Could you check a few things on this model? Use its own coordinates, in mm. A direction names the side the tool comes from. Coordinates: 2 decimals unless noted, no trailing zeros. Write each loop counter-clockwise with the first axis right and the second up, starting at its lowest first coordinate (ties: lowest second). Pieces come first, ordered by that corner, then holes. Notation, with made-up numbers: M 51,36 L 82,36 A23 cw 82,47 Z; hole C 49,-9 d2. An arc over 180 degrees is marked long. Answer as CSV lines item,"result". Start each with the question number.
Item 1: I'm going to push flat-ended pins straight in: P1, Ø3, axis at x = -5.5, z = 0, coming from the +Y side; P2, Ø2, axis at x = 0, y = 1, coming from the +Z side; P3, Ø3, axis at y = 7, z = -8, coming from the +X side; P4, Ø2.5, axis at x = 0, y = 3.5, coming from the -Z side. Where does each tip first touch, or does it pass through?
Item 2: Suppose I cut it at A-A, the plane y = 5. Write out the boundary of the cut face in (x, z).
Item 3: On a 3-axis mill with a long thin cutter (end or side, diameter ignored), from which of +Z, -Z, +X, -X, +Y, -Y can I reach the whole of each face in a straight line? I mean faces 5 (the cylindrical face through (4.28, 7.77, -0.27)), 6 (the flat face through (1.3, 3.2, 8.3)), 7 (the flat face through (-8, 7, -5)). Say none if no direction works.
Item 4: If I drill on line 1 along X through (y, z) = (7.75, 0); line 2 along Y through (x, z) = (7.5, 4.25); line 3 along X through (y, z) = (0.6, 0), over which ranges is the centre line in solid material (lowest first)? Write a range as [from, to].
Item 5: We'd pull the mould along Y, two halves only. Please class faces 1 (the cylindrical face through (8.054, 5.462, 1.788)), 2 (the flat face through (-4, 0, 0)), 3 (the cylindrical face through (-6.3, 7.51, -8.21)), 4 (the cylindrical face through (8.054, 2.362, 1.788)): +Y half, -Y half, draft (parallel to the pull), parting line (faces both ways), or undercut.
Item 6: Suppose I cut it at B-B, the plane z = 0. State how many separate pieces and enclosed holes the cut face has, and give its area (3 significant figures).
```python
from build123d import *

# Parameters (mm, degrees)
SKETCH_1_R          = 11
EXTRUDE_1_DEPTH     = 9
SKETCH_2_R          = 0.5
CUT_EXTRUDE_1_DEPTH = 18.972200756
SKETCH_3_R          = 16.549134696
SKETCH_3_R_2        = 9.25
CUT_EXTRUDE_2_DEPTH = 7
SKETCH_4_W          = 2
SKETCH_4_H          = 1.7
SKETCH_5_W          = 5
SKETCH_5_H          = 6
CUT_EXTRUDE_3_DEPTH = 7
SKETCH_6_R          = 1.4
CUT_EXTRUDE_4_DEPTH = 7
SKETCH_7_R          = 1.25
CUT_EXTRUDE_5_DEPTH = 2.5
CUT_EXTRUDE_START   = -1.5
SKETCH_8_R          = 1.25
CUT_EXTRUDE_6_DEPTH = 1.5
SKETCH_9_W          = 7
SKETCH_9_H          = 8
SKETCH_9_W_2        = 5
SKETCH_9_H_2        = 6
CUT_EXTRUDE_7_DEPTH = 2
CHAMFER_1_SIZE      = 0.5
SKETCH_10_R         = 12.5
SKETCH_10_R_2       = 10.35
CUT_EXTRUDE_8_DEPTH = 10
FILLET_1_R          = 1
SKETCH_11_R         = 1.953999565
EXTRUDE_2_DEPTH     = 2


with BuildPart() as part:
    # 草图1 → 凸台-拉伸1 (new body)
    with BuildSketch(Plane(origin=(0, 0, 0), x_dir=(1, 0, 0), z_dir=(0, 1, 0))):
        with Locations(Location((0, 0, 0), (0, 0, 270))):
            Circle(SKETCH_1_R)
    extrude(amount=EXTRUDE_1_DEPTH)

    # 草图2 → 切除-拉伸1 (cut, through all)
    with BuildSketch(Plane(origin=(0, 9, 0), x_dir=(1, 0, 0), z_dir=(0, 1, 0))):
        with Locations(Location((-5.5, 0, 0), (0, 0, 270))):
            Circle(SKETCH_2_R)
        with Locations(Location((5.5, 0, 0), (0, 0, 270))):
            Circle(SKETCH_2_R)
    extrude(amount=-CUT_EXTRUDE_1_DEPTH, mode=Mode.SUBTRACT)

    # 草图3 → 切除-拉伸2 (cut)
    with BuildSketch(Plane.XZ):
        Circle(SKETCH_3_R)
        with Locations(Location((0, 0, 0), (0, 0, 270))):
            Circle(SKETCH_3_R_2, mode=Mode.SUBTRACT)
    extrude(amount=-CUT_EXTRUDE_2_DEPTH, mode=Mode.SUBTRACT)

    # 草图4 → 切除-旋转1 (revolve, cut)
    with BuildSketch(Plane.XY, mode=Mode.PRIVATE) as cut_revolve_1_sk:
        with Locations((-9.25, 5.45)):
            Rectangle(SKETCH_4_W, SKETCH_4_H)
        with Locations((-9.25, 2.35)):
            Rectangle(SKETCH_4_W, SKETCH_4_H)
    revolve(cut_revolve_1_sk.sketch.rotate(Axis((0, 0, 0), (0, 1, 0)), 270), axis=Axis((0, 0, 0), (0, 1, 0)), mode=Mode.SUBTRACT)

    # 草图5 → 切除-拉伸3 (cut)
    with BuildSketch(Plane.XZ):
        Rectangle(SKETCH_5_W, SKETCH_5_H)
    extrude(amount=-CUT_EXTRUDE_3_DEPTH, mode=Mode.SUBTRACT)

    # 草图6 → 切除-拉伸4 (cut)
    with BuildSketch(Plane(origin=(0, 9, 0), x_dir=(1, 0, 0), z_dir=(0, 1, 0))):
        with Locations(Location((0, 0, 0), (0, 0, 270))):
            Circle(SKETCH_6_R)
    extrude(amount=-CUT_EXTRUDE_4_DEPTH, mode=Mode.SUBTRACT)

    # 草图7 → 切除-拉伸5 (cut)
    with BuildSketch(Plane(origin=(0, 9, 0), x_dir=(1, 0, 0), z_dir=(0, 1, 0))):
        with Locations(Location((-5.5, 0, 0), (0, 0, 270))):
            Circle(SKETCH_7_R)
        with Locations(Location((5.5, 0, 0), (0, 0, 270))):
            Circle(SKETCH_7_R)
    extrude(amount=-CUT_EXTRUDE_5_DEPTH, mode=Mode.SUBTRACT)

    # 草图8 → 切除-拉伸6 (cut)
    with BuildSketch(Plane.XZ.offset(CUT_EXTRUDE_START)):
        with Locations(Location((-5.5, 0, 0), (0, 0, 90))):
            Circle(SKETCH_8_R)
        with Locations(Location((5.5, 0, 0), (0, 0, 90))):
            Circle(SKETCH_8_R)
    extrude(amount=CUT_EXTRUDE_6_DEPTH, mode=Mode.SUBTRACT)

    # 草图9 → 切除-拉伸7 (cut)
    with BuildSketch(Plane.XZ):
        Rectangle(SKETCH_9_W, SKETCH_9_H)
        Rectangle(SKETCH_9_W_2, SKETCH_9_H_2, mode=Mode.SUBTRACT)
    extrude(amount=-CUT_EXTRUDE_7_DEPTH, mode=Mode.SUBTRACT)

    # 倒角1
    chamfer_1_edges = [part.edges().sort_by_distance(p)[0] for p in [
        (0, 0, 9.25),
    ]]
    chamfer(chamfer_1_edges, length=CHAMFER_1_SIZE)

    # 草图10 → 切除-拉伸8 (cut)
    with BuildSketch(Plane(origin=(0, 9, 0), x_dir=(1, 0, 0), z_dir=(0, 1, 0))):
        Circle(SKETCH_10_R)
        with Locations(Location((0, 0, 0), (0, 0, 270))):
            Circle(SKETCH_10_R_2, mode=Mode.SUBTRACT)
    extrude(amount=-CUT_EXTRUDE_8_DEPTH, mode=Mode.SUBTRACT)

    # 圆角1
    fillet_1_edges = [part.edges().sort_by_distance(p)[0] for p in [
        (0, 9, -10.35),
    ]]
    fillet(fillet_1_edges, radius=FILLET_1_R)

    # 草图11 → 凸台-拉伸2 (add)
    with BuildSketch(Plane(origin=(0, 9, 0), x_dir=(1, 0, 0), z_dir=(0, 1, 0))):
        Circle(SKETCH_11_R)
    extrude(amount=-EXTRUDE_2_DEPTH)


solid = part.part
```
Ans:
1,P1,"stops at y = 9"
1,P2,"stops at z = 9.25"
1,P3,"stops at x = 8.05"
1,P4,"stops at z = -9.25"
2,outline,"C 0,0 d16.5; hole C -5.5,0 d1; hole M -2.5,-3 L 2.5,-3 L 2.5,3 L -2.5,3 Z; hole C 5.5,0 d1"
3,face 5,"+Y"
3,face 6,"none"
3,face 7,"-Y"
4,line 1,"x = [-10.35, -6.75], [-4.25, 4.25], [6.75, 10.35]"
4,line 2,"y = [0, 1.5], [3.2, 4.6], [6.3, 9]"
4,line 3,"x = [-9.25, -6.75], [-4.25, -3.5], [3.5, 4.25], [6.75, 9.25]"
5,face 1,"undercut"
5,face 2,"-Y half"
5,face 3,"draft"
5,face 4,"undercut"
6,separate pieces,"3"
6,enclosed holes,"0"
6,area,"94.4 mm^2"
